from build123d import *

# Parameters (mm, degrees)
BOSS_EXTRUDE1_DEPTH = 1.5
FILLET1_R           = 4
SKETCH2_R           = 1
CUT_EXTRUDE1_DEPTH  = 11.5


with BuildPart() as part:
    # Sketch1 → Boss-Extrude1 (new body)
    with BuildSketch(Plane(origin=(0, 0, 0), x_dir=(1, 0, 0), z_dir=(0, 1, 0))):
        with BuildLine():
            Line((21.165401421, 16.688429867), (30.665401421, 16.688429867))
            ThreePointArc((30.665401421, 16.688429867), (37.78790042, 19.188429867), (30.665401421, 21.688429867))
            Line((30.665401421, 21.688429867), (21.165401421, 21.688429867))
            ThreePointArc((21.165401421, 21.688429867), (14.799770492, 18.961430624), (12.175333046, 12.552834047))
            Line((12.175333046, 12.552834047), (17.175333046, 12.552834047))
            ThreePointArc((17.175333046, 12.552834047), (18.33546909, 15.426150877), (21.165401421, 16.688429867))
        make_face()
        with BuildLine():
            ThreePointArc((8.055333046, 2.670166466), (10.968612985, 3.876886527), (12.175333046, 6.790166466))
            Line((12.175333046, 6.790166466), (12.175333046, 12.552834047))
            Line((12.175333046, 12.552834047), (17.175333046, 12.552834047))
            Line((17.175333046, 12.552834047), (17.175333046, 3.552834047))
            Line((17.175333046, 3.552834047), (11.122498999, -2.5))
            Line((11.122498999, -2.5), (3.122498999, -2.5))
            ThreePointArc((3.122498999, -2.5), (-3.99844492, -0.111526763), (2.978289953, 2.670166466))
            Line((2.978289953, 2.670166466), (8.055333046, 2.670166466))
        make_face()
    extrude(amount=BOSS_EXTRUDE1_DEPTH)

    # Fillet1
    fillet1_edges = [part.edges().sort_by_distance(p)[0] for p in [
        (17.175333046, 0.75, -3.552834047),
        (11.122498999, 0.75, 2.5),
    ]]
    fillet(fillet1_edges, radius=FILLET1_R)

    # Sketch2 → Cut-Extrude1 (cut)
    with BuildSketch(Plane(origin=(0, 1.5, 0), x_dir=(1, 0, 0), z_dir=(0, 1, 0))):
        Circle(SKETCH2_R)
        with Locations((33.78790042, 19.188429867)):
            Circle(SKETCH2_R)
    extrude(amount=-CUT_EXTRUDE1_DEPTH, mode=Mode.SUBTRACT)


solid = part.part
CAD build for the part. Positions are in the model's coordinates, mm. A direction names the side the tool comes from. Coordinates: 2 decimals unless noted, no trailing zeros. Loops run counter-clockwise (first coordinate to the right, second up) from the corner with the lowest first, then second, coordinate; pieces in that order, holes last. Notation, with made-up numbers: (54, 32.25) -> (104, 32.25) arc R10 cw to (104, 42.25) -> close; hole circle Ø2 at (17.25, -37). An arc over 180 degrees is marked (long way). One line per item, written item: value.
1. Slice it at B-B on z = 0. Write the cut outline in (x, y).
Answers:
outline: (-4, 0) -> (-1, 0) -> (-1, 1.5) -> (-4, 1.5) -> close; (1, 0) -> (13.62, 0) -> (13.62, 1.5) -> (1, 1.5) -> close
2. Slice it at D-D on x = 26.5. Write the cut outline in (y, z), and give its area (3 significant figures).
Answers:
outline: (0, -21.69) -> (1.5, -21.69) -> (1.5, -16.69) -> (0, -16.69) -> close
area: 7.50 mm^2
3. Pull direction X, two halves, no side cores. Call faces 1 (the face through (10.94, 0.74, -3.85)), 2 (the face through (16.862, 0.76, -3.659)), 3 (the face through (15, 0, -10)): pulls with the +X half, pulls with the -X half, needs draft (parallel to the pull), parting line crosses it, or undercut.
Answers:
face 1: undercut
face 2: pulls with the +X half
face 3: needs draft
4. Slice it at A-A on x = 0. Write the cut outline in (y, z), and give its area (3 significant figures).
Answers:
outline: (0, -4) -> (1.5, -4) -> (1.5, -1) -> (0, -1) -> close; (0, 1) -> (1.5, 1) -> (1.5, 4) -> (0, 4) -> close
area: 9.00 mm^2
5. Drill centre lines: line 1 (Z direction, x = 0, y = 1); line 2 (Z direction, x = 8, y = 0.2); line 3 (X direction, y = 0.75, z = -0.25). Where is each one in solid material? Low to high. Write a range as [from, to].
Answers:
line 1: z = [-4, -1], [1, 4]
line 2: z = [-2.67, 2.5]
line 3: x = [-3.99, -0.97], [0.97, 13.87]
6. Slice it at C-C on y = 0.9. Write the cut outline in (x, z).
Answers:
outline: (2.98, -2.67) -> (8.06, -2.67) arc R4.12 cw to (12.18, -6.79) -> (12.18, -12.55) arc R9.14 ccw to (21.17, -21.69) -> (30.67, -21.69) arc R4 ccw (long way) to (30.67, -16.69) -> (21.17, -16.69) arc R4.14 cw to (17.18, -12.55) -> (17.18, -5.21) arc R4 ccw to (16, -2.38) -> (12.29, 1.33) arc R4 ccw to (9.47, 2.5) -> (3.12, 2.5) arc R4 ccw (long way) to start; hole circle Ø2 at (0, 0); hole circle Ø2 at (33.79, -19.19)
7. Which spindle directions (+Z, -Z, +X, -X, +Y, -Y) get a long thin tool onto all of the face, cutting with end or side? Do faces 4 (the face through (33.051, 0.76, -19.864)), 5 (the face through (5, 1, -2.67)), 6 (the face through (26, 1, -16.688)), 7 (the face through (12.175, 1, -10)), 8 (the face through (6, 1, 2.5)). Say none if no direction does.
Answers:
face 4: +Y, -Y
face 5: -Z, +Y, -Y
face 6: +Z, +Y, -Y
face 7: -Z, -X, +Y, -Y
face 8: +Z, +X, +Y, -Y
